from build123d import *

# Parameters (mm, degrees)
SKETCH1_W           = 30
SKETCH1_H           = 8
SKETCH1_R           = 1.75
BOSS_EXTRUDE1_DEPTH = 2
SKETCH2_R           = 1.75
BOSS_EXTRUDE2_DEPTH = 8
FILLET1_R           = 2
SKETCH3_R           = 1.75
CUT_EXTRUDE1_DEPTH  = 7.5
CUT_EXTRUDE2_DEPTH  = 3


with BuildPart() as part:
    # Sketch1 → Boss-Extrude1 (new body)
    with BuildSketch(Plane(origin=(0, 0, 0), x_dir=(1, 0, 0), z_dir=(0, 1, 0))):
        Rectangle(SKETCH1_W, SKETCH1_H)
        with Locations((-1, -0.5)):
            Circle(SKETCH1_R, mode=Mode.SUBTRACT)
    extrude(amount=BOSS_EXTRUDE1_DEPTH)

    # Sketch2 → Boss-Extrude2 (add)
    with BuildSketch(Plane.XY.offset(4)):
        Polygon((-15, 0), (-5, 0), (5, 0), (15, 0), (15, -6.5), (-15, -6.5), align=None)
        with Locations((-10, -3)):
            Circle(SKETCH2_R, mode=Mode.SUBTRACT)
        with Locations((10, -3)):
            Circle(SKETCH2_R, mode=Mode.SUBTRACT)
    extrude(amount=-BOSS_EXTRUDE2_DEPTH)

    # Fillet1
    fillet1_edges = [part.edges().sort_by_distance(p)[0] for p in [
        (-15, -2.25, -4),
        (15, -2.25, -4),
    ]]
    fillet(fillet1_edges, radius=FILLET1_R)

    # Sketch3 → Cut-Extrude1 (cut, through all)
    with BuildSketch(Plane(origin=(0, 0, 0), x_dir=(1, 0, 0), z_dir=(0, 1, 0))):
        with Locations((-1, -0.5)):
            Circle(SKETCH3_R)
    extrude(amount=-CUT_EXTRUDE1_DEPTH, mode=Mode.SUBTRACT)

    # Sketch4 → Cut-Extrude2 (cut)
    with BuildSketch(Plane.XZ.offset(6.5)):
        Polygon((2.464101615, 0.5), (0.732050808, 3.5), (-2.732050808, 3.5), (-4.464101615, 0.5), (-2.732050808, -2.5), (0.732050808, -2.5), align=None)
    extrude(amount=-CUT_EXTRUDE2_DEPTH, mode=Mode.SUBTRACT)


solid = part.part
Geometry: final body of the model. Coordinates: model frame, mm. A direction names the side the tool comes from. Coordinates: 2 decimals unless noted, no trailing zeros. Order: outer loops, then holes, each group sorted by start corner. A loop starts at its lowest first (then second) coordinate and runs counter-clockwise, first axis right, second up.
(1) Section query D-D (x = 10). Return the cut outline in (y, z), plus the area to 3 significant figures.
(2) First-contact query: pin 1 (3 mm diameter, centred on x = -1, z = 1, fed in from -Y). Flat tip, straight axial feed; report the tip coordinate or a pass-through.
(3) Access query for faces 5 (the face through (0, -2, -4)), 6 (the face through (0.5, -3.5, -0.8)). Directions: +Z, -Z, +X, -X, +Y, -Y. A direction counts if a zero-diameter tool reaches every point of the face in a straight line with its end or side. Return the directions, or none.
(4) Section query B-B (y = -3). Return the cut outline in (x, z).
(5) Material intervals for probe 1 along Y at (x, z) = (-10, 2.5); probe 2 along X at (y, z) = (1.05, 0.5); probe 3 along Z at (x, y) = (0.5, -5.25), sorted ascending.
(6) Section query A-A (x = -1). Return the cut outline in (y, z), plus the area to 4 significant figures.
(7) Section query C-C (z = -3). Return the cut outline in (x, y), plus the area to 3 significant figures.
(8) Draft query along Z for faces 1 (the face through (0, -2, 4)), 2 (the face through (-3.6, -5, 2)), 3 (the face through (-15, -2, 1)), 4 (the face through (-14.4, -2.31, -3.43)). Return one class per face: pulls with the +Z half, pulls with the -Z half, needs draft (parallel to the pull), parting line crosses it, or undercut.
Solution:
1. outline: (-6.5, -4) - (-4.75, -4) - (-4.75, 4) - (-6.5, 4) - close; (-1.25, -4) - (2, -4) - (2, 4) - (-1.25, 4) - close
1. area: 40.0 mm2
2. pin 1: stops at y = -3.5
3. face 5: -Z, +X, -X, +Y, -Y
3. face 6: -Y
4. outline: (-15, -2) arc R2 ccw to (-13, -4) - (-11.75, -4) - (-11.75, 4) - (-15, 4) - close; (-8.25, -4) - (8.25, -4) - (8.25, 4) - (-8.25, 4) - close; (11.75, -4) - (13, -4) arc R2 ccw to (15, -2) - (15, 4) - (11.75, 4) - close; hole circle Ø3.5 at (-1, 0.5)
5. probe 1: y = -6.5 to -4.75, -1.25 to 2
5. probe 2: x = -15 to -2.75, 0.75 to 15
5. probe 3: z = -4 to -2.5, 3.5 to 4
6. outline: (-6.5, -4) - (2, -4) - (2, -1.25) - (-3.5, -1.25) - (-3.5, -2.5) - (-6.5, -2.5) - close; (-6.5, 3.5) - (-3.5, 3.5) - (-3.5, 2.25) - (2, 2.25) - (2, 4) - (-6.5, 4) - close
6. area: 30.75 mm2
7. outline: (-14.73, -6.5) - (14.73, -6.5) - (14.73, 2) - (-14.73, 2) - close; hole circle Ø3.5 at (-10, -3); hole circle Ø3.5 at (10, -3)
7. area: 231 mm2
8. face 1: pulls with the +Z half
8. face 2: undercut
8. face 3: needs draft
8. face 4: pulls with the -Z half
